```python
from build123d import *

# Parameters (mm, degrees)
F0_W     = 304.8
F0_H     = 88.9
F1_DEPTH = 6.35
F2_W     = 15.24
F2_H     = 15.24
F3_DEPTH = 25.4
F5_D     = 4.318


with BuildPart() as f1:
    # F0 (on Top) → F1 (new body)
    with BuildSketch(Plane.XY):
        Rectangle(F0_W, F0_H)
    extrude(amount=-F1_DEPTH)

    # F2 (on face) → F3 (cut)
    with BuildSketch(Plane.XY):
        with Locations((-80.9625, -31.75)):
            Rectangle(F2_W, F2_H)
        with Locations((80.9625, -31.75)):
            Rectangle(F2_W, F2_H)
    extrude(amount=-F3_DEPTH, mode=Mode.SUBTRACT)

    # F5 (through all)
    with Locations(Plane.XY):
        with Locations((-50.9905, 39.878), (-139.8905, 17.272), (-50.9905, 1.778), (-139.8905, -20.828), (139.8905, 1.778), (139.8905, 39.878), (50.9905, 17.272), (50.9905, -20.828)):
            Hole(F5_D / 2)


solid = f1.part
```
Input: part model. Units: mm. Frame: model coordinates. A direction names the side the tool comes from. Round coordinates to 2 decimals unless told otherwise and drop trailing zeros. Loops run counter-clockwise (first coordinate to the right, second up) from the corner with the lowest first, then second, coordinate; pieces in that order, holes last. Notation, with made-up numbers: (1, 9) -> (52, 9) arc R20 cw to (52, 43) -> close; hole circle Ø10 at (7, -16.5). An arc over 180 degrees is marked (long way). One line per item, written item: value.
(1) Section A-A (x = 80.5). Return the cut outline in (y, z).
Geometry check:
outline: (-44.45, -6.35) -> (-39.37, -6.35) -> (-39.37, 0) -> (-44.45, 0) -> close; (-24.13, -6.35) -> (44.45, -6.35) -> (44.45, 0) -> (-24.13, 0) -> close
(2) Set-up query: faces 4 (the face through (-2, 44.45, -3)), 5 (the face through (81, -39.37, -3)). Return all of +Z, -Z, +X, -X, +Y, -Y with unobstructed straight access to the full face (end or side cutting, diameter ignored); none if empty.
Geometry check:
face 4: +Z, -Z, +X, -X, +Y
face 5: +Z, -Z
(3) Pin query (flat end, axial travel): pin 1 (3.5 mm diameter, centred on x = 139.89, y = 39.88, fed in from +Z). Return the tip coordinate at first contact, or that it passes through.
Geometry check:
pin 1: through
(4) Material intervals for line 1 (X direction, y = -20.5, z = -5.75); line 2 (X direction, y = 1.5, z = -3.25); line 3 (Y direction, x = -76.5, z = -4.5), sorted ascending. Write a range as [from, to].
Geometry check:
line 1: [-152.4, -142.02], [-137.76, 48.86], [53.12, 152.4]
line 2: [-152.4, -53.13], [-48.85, 137.75], [142.03, 152.4]
line 3: [-44.45, -39.37], [-24.13, 44.45]
(5) Section B-B (y = -33). Return the cut outline in (x, z).
Geometry check:
outline: (-152.4, -6.35) -> (-88.58, -6.35) -> (-88.58, 0) -> (-152.4, 0) -> close; (-73.34, -6.35) -> (73.34, -6.35) -> (73.34, 0) -> (-73.34, 0) -> close; (88.58, -6.35) -> (152.4, -6.35) -> (152.4, 0) -> (88.58, 0) -> close
(6) Mould query, pull axis X, two halves, no side actions, for faces 1 (the face through (88.583, -32, -3)), 2 (the face through (-2, 1, -6.35)), 3 (the face through (-152.4, -1, -3)). Classes: pulls with the +X half, pulls with the -X half, needs draft (parallel to the pull), parting line crosses it, or undercut.
Geometry check:
face 1: undercut
face 2: needs draft
face 3: pulls with the -X half
(7) Section C-C (z = -5). Give the number of separate pieces and of enclosed holes in the cut face, plus the area to 3 significant figures.
Geometry check:
separate pieces: 1
enclosed holes: 10
area: 26,500 mm2
